Verification items for the finished model (mm, model axes). Face numbers are marked on the shaded views. A direction names the side the tool comes from. Give positions to 0.01 mm unless a question says otherwise; leave off trailing zeros. Write each loop counter-clockwise with the first axis right and the second up, starting at its lowest first coordinate (ties: lowest second). Pieces come first, ordered by that corner, then holes. Notation, with made-up numbers: M 15.5,38 L 50.5,38 A32 cw 50.5,74 Z; hole C 9.5,-2 d4. An arc over 180 degrees is marked long. Answer as a JSON object with one key per item and string values.
Autodesk Inventor part; units mm, degrees
ref_plane "YZ Plane" through (0, 0, 0) normal (1, 0, 0) x (0, 1, 0)
ref_plane "XZ Plane" through (0, 0, 0) normal (0, 1, 0) x (-1, 0, 0)
ref_plane "XY Plane" through (0, 0, 0) normal (0, 0, 1) x (1, 0, 0)
sketch "Sketch1" plane through (0, 0, 0) normal (0, 1, 0) x (-1, 0, 0)
  point P0 (0, 0)
sketch "Sketch2" plane through (0, 0, 0) normal (0, 1, 0) x (-1, 0, 0)
  line L0 (0, 0) -> (15.2, 0)
  line L1 (15.2, 0) -> (15.2, -7.2)
  line L2 (15.2, -7.2) -> (0, -7.2)
  line L3 (0, -7.2) -> (0, 0)
  dimension "d0" = 15.2
  dimension "d1" = 7.2
extrude "Extrusion1" add sketch "Sketch2" along normal blind 7.7
fillet "Fillet1" radius 3.6 2 edges at (0, 3.85, 0) (0, 3.85, -7.2)
fillet "Fillet2" radius 3.6 2 edges at (-15.2, 3.85, 0) (-15.2, 3.85, -7.2)
sketch "Sketch3" plane through (0, 7.7, 0) normal (0, 1, 0) x (1, 0, 0)
  arc A0 (-3.6, 0) -> (-3.6, 7.2) centre (-3.6, 3.6) ccw
  line L0 (0, 3.6) -> (-1, 3.6)
  line L1 (-1, 3.6) -> (-1, 4.5)
  line L2 (-1, 3.6) -> (-1, 2.7)
  line L3 (-1, 4.5) -> (-5.8, 4.5)
  line L4 (-5.8, 4.5) -> (-5.8, 2.7)
  line L5 (-5.8, 2.7) -> (-1, 2.7)
  line L6 (-1, 2.7) -> (-1, 4.5)
  line L7 (-1, 3.6) -> (-3.4, 3.6)
  line L8 (-3.4, 3.6) -> (-3.4, 6)
  line L9 (-3.4, 3.6) -> (-3.4, 1.2)
  line L10 (-3.4, 6) -> (-2.5, 6)
  line L11 (-3.4, 6) -> (-4.3, 6)
  line L12 (-4.3, 6) -> (-2.5, 6)
  line L13 (-2.5, 6) -> (-2.5, 1.2)
  line L14 (-2.5, 1.2) -> (-4.3, 1.2)
  line L15 (-4.3, 1.2) -> (-4.3, 6)
  point P0 (0, 0)
  point P1 (-4.3, 2.7)
  point P2 (-4.3, 4.5)
  point P3 (-2.5, 4.5)
  point P4 (-3.4, 4.5)
  point P5 (-2.5, 2.7)
  point P6 (-3.4, 2.7)
  dimension "d6" = 1
  dimension "d14" = 0.9
  dimension "d15" = 0.9
  dimension "d16" = 4.8
  dimension "d17" = 2.4
  dimension "d18" = 2.4
  dimension "d19" = 0.9
  dimension "d20" = 0.9
  dimension "d21" = 4.8
extrude "Extrusion2" cut sketch "Sketch3" against normal through all contours L15 L5 L4 L3
extrude "Extrusion3" cut sketch "Sketch3" against normal through all contours L3 L8 L10 L13
extrude "Extrusion4" cut sketch "Sketch3" against normal through all contours L3 L15 L11 L8
extrude "Extrusion5" cut sketch "Sketch3" against normal through all contours L13 L14 L9 L5
extrude "Extrusion6" cut sketch "Sketch3" against normal through all contours L9 L14 L15 L5
extrude "Extrusion7" cut sketch "Sketch3" against normal through all contours L7 L13 L3 L1 | L2 L5 L13 L7 | L13 L5 L9 L7 | L7 L8 L3 L13 | L9 L5 L15 L3 L8 | L15 L5 L4 L3
fillet "Fillet3" radius 0.2 1 edges at (-4.3, 3.85, -4.5)
fillet "Fillet4" radius 0.2 1 edges at (-4.3, 3.85, -2.7)
fillet "Fillet5" radius 0.2 1 edges at (-2.5, 3.85, -2.7)
fillet "Fillet6" radius 0.2 1 edges at (-2.5, 3.85, -4.5)
sketch "Sketch4" plane through (0, 7.7, 0) normal (0, 1, 0) x (1, 0, 0)
  arc A0 (-11.6, 7.2) -> (-11.6, 0) centre (-11.6, 3.6) ccw
  line L0 (-15.2, 3.6) -> (-14, 3.6)
  line L1 (-14, 3.6) -> (-10.3, 3.6)
  circle A1 centre (-12.15, 3.6) radius 1.85
  point P0 (0, 0)
  dimension "d38" = 1.2
  dimension "d39" = 3.7
extrude "Extrusion8" cut sketch "Sketch4" against normal through all
sketch "Sketch5" plane through (-3.6, 0, 0) normal (0, 0, 1) x (1, 0, 0)
  line L0 (-6.2992, 6.9034) -> (0.3672, 6.9034) construction
  line L1 (0.3672, 6.9034) -> (0.3672, 0.2653) construction
  line L2 (0.3672, 0.2653) -> (-6.2992, 0.2653) construction
  line L3 (-6.2992, 0.2653) -> (-6.2992, 6.9034) construction
  spline S0 degree 2 poles (-1.5438, 2.6769) (-1.5438, 2.2221) (-1.8898, 1.5251) (-2.1766, 1.2977) knots 0 0 0 1 2 2 2
  spline S1 degree 2 poles (-2.1766, 1.2977) (-2.5226, 1.0308) (-3.3086, 0.8034) (-3.9314, 0.8034) knots 0 0 0 1 2 2 2
  line L4 (-3.9314, 0.8034) -> (-5.6813, 0.8034)
  line L5 (-5.6813, 0.8034) -> (-5.6813, 6.9034)
  line L6 (-5.6813, 6.9034) -> (-4.0649, 6.9034)
  spline S2 degree 2 poles (-4.0649, 6.9034) (-3.4124, 6.9034) (-2.7599, 6.8193) (-2.4633, 6.6562) knots 0 0 0 1 2 2 2
  spline S3 degree 2 poles (-2.4633, 6.6562) (-2.1321, 6.4832) (-1.8305, 5.9147) (-1.8305, 5.5292) knots 0 0 0 1 2 2 2
  spline S4 degree 2 poles (-1.8305, 5.5292) (-1.8305, 5.0991) (-2.2853, 4.4169) (-2.6857, 4.2241) knots 0 0 0 1 2 2 2
  line L7 (-2.6857, 4.2241) -> (-2.6857, 4.1945)
  spline S5 degree 2 poles (-2.6857, 4.1945) (-2.142, 4.0462) (-1.5438, 3.2602) (-1.5438, 2.6769) knots 0 0 0 1 2 2 2
  spline S6 degree 2 poles (-2.3891, 2.6423) (-2.3891, 2.9883) (-2.5868, 3.4332) (-2.8834, 3.5914) knots 0 0 0 1 2 2 2
  spline S7 degree 2 poles (-2.8834, 3.5914) (-3.0762, 3.6903) (-3.531, 3.7496) (-3.9512, 3.7496) knots 0 0 0 1 2 2 2
  line L8 (-3.9512, 3.7496) -> (-4.8706, 3.7496)
  line L9 (-4.8706, 3.7496) -> (-4.8706, 1.4954)
  line L10 (-4.8706, 1.4954) -> (-4.2132, 1.4954)
  spline S8 degree 2 poles (-4.2132, 1.4954) (-3.6793, 1.4954) (-3.0663, 1.5943) (-2.8291, 1.7525) knots 0 0 0 1 2 2 2
  spline S9 degree 2 poles (-2.8291, 1.7525) (-2.6017, 1.9156) (-2.3891, 2.321) (-2.3891, 2.6423) knots 0 0 0 1 2 2 2
  spline S10 degree 2 poles (-2.6758, 5.4155) (-2.6758, 5.633) (-2.8241, 5.9592) (-2.9873, 6.0531) knots 0 0 0 1 2 2 2
  spline S11 degree 2 poles (-2.9873, 6.0531) (-3.185, 6.1619) (-3.6645, 6.2113) (-4.0945, 6.2113) knots 0 0 0 1 2 2 2
  line L11 (-4.0945, 6.2113) -> (-4.8706, 6.2113)
  line L12 (-4.8706, 6.2113) -> (-4.8706, 4.4268)
  line L13 (-4.8706, 4.4268) -> (-3.9512, 4.4268)
  spline S12 degree 2 poles (-3.9512, 4.4268) (-3.5706, 4.4268) (-3.2097, 4.5059) (-3.0169, 4.6295) knots 0 0 0 1 2 2 2
  spline S13 degree 2 poles (-3.0169, 4.6295) (-2.8291, 4.7481) (-2.6758, 5.1287) (-2.6758, 5.4155) knots 0 0 0 1 2 2 2
  point P0 (3.6, 0)
extrude "Extrusion9" cut sketch "Sketch5" against normal blind 0.2
sketch "Sketch6" plane through (0, 7.7, 0) normal (0, 1, 0) x (1, 0, 0)
  circle A0 centre (-12.15, 3.6) radius 1.85
  circle A1 centre (-12.15, 3.6) radius 1.95
  point P0 (0, 0)
  dimension "d44" = 3.9
extrude "Extrusion10" cut sketch "Sketch6" against normal through all
sketch "Sketch7" plane through (0, 7.7, 0) normal (0, 1, 0) x (1, 0, 0)
  line L0 (-4.3, 4.5) -> (-4.7532, 4.5)
  line L1 (-4.7532, 4.5) -> (-4.7532, 4.9695)
  line L2 (-4.7532, 4.9695) -> (-4.3, 4.9695)
  line L3 (-4.3, 4.9695) -> (-4.3, 4.5)
  arc A0 (-2.5, 4.7) -> (-2.3, 4.5) centre (-2.3, 4.7) ccw
  line L4 (-2.3, 4.7) -> (-2.5, 4.7)
  line L5 (-2.5, 4.7) -> (-2.5, 4.5)
  line L6 (-2.5, 4.5) -> (-2.3, 4.5)
  line L7 (-2.3, 4.5) -> (-2.3, 4.7)
  arc A1 (-2.3, 2.7) -> (-2.5, 2.5) centre (-2.3, 2.5) ccw
  line L8 (-2.3, 2.5) -> (-2.5, 2.5)
  line L9 (-2.5, 2.5) -> (-2.5, 2.7)
  line L10 (-2.5, 2.7) -> (-2.3, 2.7)
  line L11 (-2.3, 2.7) -> (-2.3, 2.5)
  arc A2 (-4.3, 2.5) -> (-4.5, 2.7) centre (-4.5, 2.5) ccw
  line L12 (-4.5, 2.5) -> (-4.3, 2.5)
  line L13 (-4.3, 2.5) -> (-4.3, 2.7)
  line L14 (-4.3, 2.7) -> (-4.5, 2.7)
  line L15 (-4.5, 2.7) -> (-4.5, 2.5)
  point P0 (0, 0)
extrude "Extrusion11" add sketch "Sketch7" against normal blind 7.7 contours L0 L1 L2 L3
extrude "Extrusion12" add sketch "Sketch7" against normal blind 7.7 contours L4 L7 A0 | A0 L6 L5
extrude "Extrusion13" add sketch "Sketch7" against normal blind 7.7 contours L12 L15 A2 | A2 L14 L13
extrude "Extrusion14" add sketch "Sketch7" against normal blind 7.7 contours L11 L8 A1 | A1 L9 L10
sketch "Sketch8" plane through (0, 7.7, 0) normal (0, 1, 0) x (1, 0, 0)
  line L0 (-2.5, 2.7) -> (-1, 2.7)
  line L1 (-4.3, 1.2) -> (-2.5, 1.2)
  line L2 (-2.5, 2.7) -> (-2.7, 2.7)
  line L3 (-2.7, 2.7) -> (-2.7, 1.2)
  line L4 (-2.7, 1.2) -> (-2.5, 1.2)
  line L5 (-2.5, 1.2) -> (-2.5, 2.7)
  line L6 (-2.5, 6) -> (-4.3, 6)
  line L7 (-2.5, 6) -> (-2.7, 6)
  line L8 (-2.7, 6) -> (-2.7, 4.4977)
  line L9 (-2.7, 4.4977) -> (-2.5, 4.4977)
  line L10 (-2.5, 4.4977) -> (-2.5, 6)
  line L11 (-4.3, 4.5) -> (-5.8, 4.5)
  line L12 (-5.8, 4.5) -> (-6, 4.5)
  line L13 (-6, 4.5) -> (-6, 2.7)
  line L14 (-6, 2.7) -> (-5.8, 2.7)
  line L15 (-5.8, 2.7) -> (-5.8, 4.5)
  line L16 (-4.3, 6) -> (-4.5, 6)
  line L17 (-4.5, 6) -> (-4.5, 4.5)
  line L18 (-4.5, 4.5) -> (-4.3, 4.5)
  line L19 (-4.3, 4.5) -> (-4.3, 6)
  line L20 (-4.3, 2.7) -> (-4.3, 1.2)
  line L21 (-4.3, 2.7) -> (-4.5, 2.7)
  line L22 (-4.5, 2.7) -> (-4.5, 1.2)
  line L23 (-4.5, 1.2) -> (-4.3, 1.2)
  line L24 (-4.3, 1.2) -> (-4.3, 2.7)
  point P0 (0, 0)
  dimension "d55" = 0.2
  dimension "d56" = 0.2
  dimension "d57" = 0.2
  dimension "d58" = 0.2
  dimension "d59" = 0.2
extrude "Extrusion15" add sketch "Sketch8" against normal blind 7.7 contours L10 L9 L8 L6
extrude "Extrusion16" add sketch "Sketch8" against normal blind 7.7 contours L3 L2 L5 L1
extrude "Extrusion17" cut sketch "Sketch8" against normal through all contours L19 L11 L17 L16
extrude "Extrusion18" cut sketch "Sketch8" against normal through all contours L23 L22 L21 L20
extrude "Extrusion19" cut sketch "Sketch8" against normal through all contours L15 L14 L13 L12
sketch "Sketch9" plane through (0, 7.7, 0) normal (0, 1, 0) x (1, 0, 0)
  point P0 (0, 0)
sketch "Sketch10" plane through (0, 7.7, 0) normal (0, 1, 0) x (1, 0, 0)
  line L0 (-6, 4.5) -> (-4.5, 4.5)
  line L1 (-2.7, 2.7) -> (-2.7, 1.2)
  line L2 (-4.5, 4.5) -> (-2.7, 4.5)
  line L3 (-2.7, 4.5) -> (-2.7, 2.7)
  line L4 (-2.7, 2.7) -> (-4.5, 2.7)
  line L5 (-4.5, 2.7) -> (-4.5, 4.5)
  line L6 (-4.5, 6) -> (-2.7, 6)
  line L7 (-4.5, 6) -> (-2.7, 6)
  line L8 (-2.7, 6) -> (-2.7, 6.2)
  line L9 (-2.7, 6.2) -> (-4.5, 6.2)
  line L10 (-4.5, 6.2) -> (-4.5, 6)
  line L11 (-6, 4.5) -> (-6.2, 4.5)
  line L12 (-6.2, 4.5) -> (-6.2, 2.7)
  line L13 (-6.2, 2.7) -> (-6, 2.7)
  line L14 (-6, 2.7) -> (-6, 4.5)
  line L15 (-2.7, 1.2) -> (-4.5, 1.2)
  line L16 (-4.5, 1.2) -> (-4.5, 1)
  line L17 (-4.5, 1) -> (-2.7, 1)
  line L18 (-2.7, 1) -> (-2.7, 1.2)
  point P0 (0, 0)
  dimension "d70" = 0.2
  dimension "d71" = 0.2
  dimension "d72" = 0.2
extrude "Extrusion20" cut sketch "Sketch10" against normal through all contours L10 L9 L8 L6
extrude "Extrusion21" cut sketch "Sketch10" against normal through all contours L14 L13 L12 L11
extrude "Extrusion22" cut sketch "Sketch10" against normal through all contours L18 L17 L16 L15
fillet "Fillet7" radius 0.2 1 edges at (-4.5, 3.85, -4.5)
fillet "Fillet8" radius 0.2 1 edges at (-2.7, 3.85, -4.4977)
fillet "Fillet9" radius 0.2 1 edges at (-2.7, 3.85, -2.7)
fillet "Fillet10" radius 0.2 1 edges at (-4.5, 3.85, -2.7)
sketch "Sketch11" plane through (-3.6, 0, 0) normal (0, 0, 1) x (1, 0, 0)
  line L0 (-7.3139, 7.2702) -> (-0.5941, 7.2702)
  line L1 (-0.5941, 7.2702) -> (-0.5941, 0.3916)
  line L2 (-0.5941, 0.3916) -> (-7.3139, 0.3916)
  line L3 (-7.3139, 0.3916) -> (-7.3139, 7.2702)
  point P0 (3.6, 0)
extrude "Extrusion23" add sketch "Sketch11" against normal blind 0.5
properties part number "part1_3DPrint"
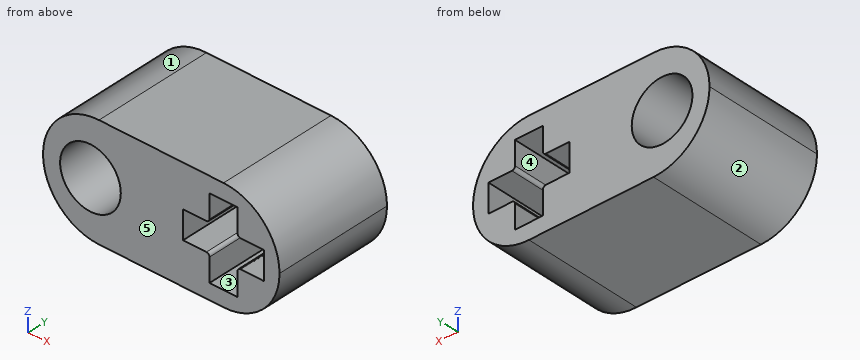
1) Section check D-D on z = -6. Record the boundary of the cut face in (x, y).
Completed:
{"outline": "M -14.28,0 L -4.5,0 L -4.5,7.7 L -14.28,7.7 Z; M -2.7,0 L -0.92,0 L -0.92,7.7 L -2.7,7.7 Z"}
2) Go/stop test with flat-tipped pins: pin 1 (1.5 mm diameter, centred on y = 1, z = -4, fed in from +X); pin 2 (1.2 mm diameter, centred on y = 2, z = -2, fed in from -X); pin 3 (1.2 mm diameter, centred on x = -2, y = 3.5, fed in from +Z); pin 4 (2 mm diameter, centred on y = 6.5, z = -6.5, fed in from +X). Record where each tip stops, or that it passes through.
Completed:
{"pin 1": "stops at x = 0", "pin 2": "stops at x = -15.06", "pin 3": "stops at z = -0.14", "pin 4": "stops at x = -0.54"}
3) Section check A-A on y = 5. Count the separate pieces of the cut face and the enclosed holes in it, and give its area (3 significant figures).
Completed:
{"separate pieces": "1", "enclosed holes": "2", "area": "70.9 mm2"}
4) Section check B-B on z = -5. Record the boundary of the cut face in (x, y).
Completed:
{"outline": "M -14.92,0 L -13.51,0 L -13.51,7.7 L -14.92,7.7 Z; M -10.79,0 L -4.5,0 L -4.5,7.7 L -10.79,7.7 Z; M -2.7,0 L -0.28,0 L -0.28,7.7 L -2.7,7.7 Z"}
5) Thickness scan on L1, parallel to X at y = 4, z = -3.6; L2, parallel to X at y = 1.25, z = -2.5; L3, parallel to Z at x = -5.75, y = 6.25. Record the ranges inside material, lowest first.
Completed:
{"L1": "x = -15.2 to -14.1, -10.2 to -6.2, -1 to 0", "L2": "x = -15.03 to -13.76, -10.54 to -4.5, -2.7 to -0.17", "L3": "z = -7.2 to -4.5, -2.7 to 0"}
6) Access from +Z, -Z, +X, -X, +Y, -Y to the whole of each face (thin tool, end or side, straight path). Record for the marked faces 4 and 5.
Completed:
{"face 4": "+Y, -Y", "face 5": "+Z, -Z, +X, -X, -Y"}
7) Release check for a two-part mould opening along Z. For the marked faces 1, 2 and 3 record: pulls with the +Z half, pulls with the -Z half, needs draft (parallel to the pull), parting line crosses it, or undercut.
Completed:
{"face 1": "pulls with the +Z half", "face 2": "pulls with the -Z half", "face 3": "undercut"}
8) Section check C-C on x = -11. Record the boundary of the cut face in (y, z), and give its area (3 significant figures).
Completed:
{"outline": "M 0,-7.2 L 7.7,-7.2 L 7.7,-5.17 L 0,-5.17 Z; M 0,-2.03 L 7.7,-2.03 L 7.7,0 L 0,0 Z", "area": "31.2 mm2"}
